Autodesk Fusion 360 part; units mm, degrees
sketch "Sketch1" plane through (0, 0, 0) normal (0, 0, 1) x (1, 0, 0)
  line L0 (0, 0) -> (74, 0)
  line L1 (74, 0) -> (74, 83)
  line L2 (74, 83) -> (0, 83)
  line L3 (0, 83) -> (0, 0)
  dimension "d1" = 74
  dimension "d2" = 83
extrude "Extrude1" add sketch "Sketch1" along normal blind 5
sketch "Sketch2" plane through (0, 0, 5) normal (0, 0, 1) x (-1, 0, 0)
  line L0 (0, -83) -> (0, 0)
  line L1 (0, 0) -> (-74, 0)
  line L2 (-74, 0) -> (-74, -83)
  line L3 (-74, -83) -> (0, -83)
  line L4 (-30.5, -77.2) -> (-71, -77.2)
  line L5 (-71, -77.2) -> (-71, -42.5)
  line L6 (-71, -42.5) -> (-30.5, -42.5)
  line L7 (-30.5, -42.5) -> (-30.5, -77.2)
  line L8 (-55.8, -22.25) -> (-67.8, -22.25)
  line L9 (-67.8, -22.25) -> (-67.8, -10.25)
  line L10 (-67.8, -10.25) -> (-55.8, -10.25)
  line L11 (-55.8, -10.25) -> (-55.8, -22.25)
  line L12 (-55.8, -35.25) -> (-67.8, -35.25)
  line L13 (-67.8, -35.25) -> (-67.8, -23.25)
  line L14 (-67.8, -23.25) -> (-55.8, -23.25)
  line L15 (-55.8, -23.25) -> (-55.8, -35.25)
  line L16 (-55.8, -29.25) -> (-67.8, -29.25) construction
  line L17 (-61.8, -35.25) -> (-61.8, -23.25) construction
  circle A0 centre (-61.8, -29.25) radius 5
  line L18 (-61.8, -22.25) -> (-61.8, -10.25) construction
  line L19 (-55.8, -16.25) -> (-67.8, -16.25) construction
  circle A1 centre (-61.8, -16.25) radius 5
  line L20 (-25.25, -10.5) -> (-13.25, -10.5)
  line L21 (-13.25, -10.5) -> (-13.25, -22.5)
  line L22 (-13.25, -22.5) -> (-25.25, -22.5)
  line L23 (-25.25, -22.5) -> (-25.25, -10.5)
  circle A2 centre (-19.25, -16.5) radius 5
  line L24 (-38.8, -4) -> (-26.8, -4)
  line L25 (-26.8, -4) -> (-26.8, -16)
  line L26 (-26.8, -16) -> (-38.8, -16)
  line L27 (-38.8, -16) -> (-38.8, -4)
  circle A3 centre (-32.8, -10) radius 5
  line L28 (-38.8, -17) -> (-26.8, -17)
  line L29 (-26.8, -17) -> (-26.8, -29)
  line L30 (-26.8, -29) -> (-38.8, -29)
  line L31 (-38.8, -29) -> (-38.8, -17)
  circle A4 centre (-32.8, -23) radius 5
  line L32 (-53, -10.5) -> (-41, -10.5)
  line L33 (-41, -10.5) -> (-41, -22.5)
  line L34 (-41, -22.5) -> (-53, -22.5)
  line L35 (-53, -22.5) -> (-53, -10.5)
  circle A5 centre (-47, -16.5) radius 5
  line L36 (-14.75, -36.25) -> (-2.75, -36.25)
  line L37 (-2.75, -36.25) -> (-2.75, -48.25)
  line L38 (-2.75, -48.25) -> (-14.75, -48.25)
  line L39 (-14.75, -48.25) -> (-14.75, -36.25)
  circle A6 centre (-8.75, -42.25) radius 5
  line L40 (-14.75, -23.25) -> (-2.75, -23.25)
  line L41 (-2.75, -23.25) -> (-2.75, -35.25)
  line L42 (-2.75, -35.25) -> (-14.75, -35.25)
  line L43 (-14.75, -35.25) -> (-14.75, -23.25)
  circle A7 centre (-8.75, -29.25) radius 5
  circle A8 centre (-25.1, -55.75) radius 2.65
  dimension "d5" = 30.5
  dimension "d6" = 42.5
  dimension "d7" = 34.7
  dimension "d8" = 40.5
  dimension "d11" = 12
  dimension "d14" = 12
  dimension "d15" = 6.2
  dimension "d16" = 10.25
  dimension "d17" = 6.2
  dimension "d19" = 1
  dimension "d20" = 10
  dimension "d21" = 10
  dimension "d22" = 12
  dimension "d23" = 10
  dimension "d24" = 12
  dimension "d25" = 10
  dimension "d26" = 12
  dimension "d27" = 10
  dimension "d28" = 12
  dimension "d29" = 10
  dimension "d32" = 10.5
  dimension "d33" = 6
  dimension "d34" = 6
  dimension "d35" = 4
  dimension "d36" = 6
  dimension "d37" = 6
  dimension "d38" = 21
  dimension "d39" = 17
  dimension "d40" = 6
  dimension "d41" = 6
  dimension "d42" = 35.2
  dimension "d43" = 6
  dimension "d44" = 6
  dimension "d45" = 13.25
  dimension "d46" = 10.5
  dimension "d47" = 12
  dimension "d48" = 10
  dimension "d49" = 6
  dimension "d50" = 6
  dimension "d51" = 12
  dimension "d52" = 10
  dimension "d53" = 6
  dimension "d54" = 6
  dimension "d55" = 2.75
  dimension "d56" = 23.25
  dimension "d57" = 1
  dimension "d58" = 5.3
  dimension "d59" = 27.25
  dimension "d60" = 25.1
extrude "Extrude3" cut sketch "Sketch2" against normal blind 5 contours A8
extrude "Extrude2" cut sketch "Sketch2" against normal blind 5 contours L4 L5 L6 L7 | A0 | A1 | A2 | A3 | A4 | A5 | A6 | A7
sketch "Sketch3" plane through (74, 0, 0) normal (1, 0, 0) x (0, 1, 0)
  line L0 (0, 0) -> (83, 0)
  line L1 (83, 0) -> (83, 5)
  line L2 (83, 5) -> (0, 5)
  line L3 (0, 5) -> (0, 0)
  line L4 (0, 5) -> (7.4455, 5)
  line L5 (7.4455, 5) -> (7.4455, 0)
  line L6 (7.4455, 0) -> (0, 0)
  line L7 (0, 0) -> (0, 5)
  line L8 (15.1109, 0) -> (15.1109, 5)
  line L9 (15.1109, 5) -> (22.5564, 5)
  line L10 (22.5564, 5) -> (22.5564, 0)
  line L11 (22.5564, 0) -> (15.1109, 0)
  line L12 (30.2218, 0) -> (30.2218, 5)
  line L13 (30.2218, 5) -> (37.6673, 5)
  line L14 (37.6673, 5) -> (37.6673, 0)
  line L15 (37.6673, 0) -> (30.2218, 0)
  line L16 (45.3327, 0) -> (45.3327, 5)
  line L17 (45.3327, 5) -> (52.7782, 5)
  line L18 (52.7782, 5) -> (52.7782, 0)
  line L19 (52.7782, 0) -> (45.3327, 0)
  line L20 (60.4436, 0) -> (60.4436, 5)
  line L21 (60.4436, 5) -> (67.8891, 5)
  line L22 (67.8891, 5) -> (67.8891, 0)
  line L23 (67.8891, 0) -> (60.4436, 0)
  line L24 (75.5545, 0) -> (75.5545, 5)
  line L25 (75.5545, 5) -> (83, 5)
  line L26 (83, 5) -> (83, 0)
  line L27 (83, 0) -> (75.5545, 0)
  dimension "d70" = 7.4455
  dimension "d74" = 75.5545
  dimension "d75" = 0
extrude "Extrude4" add sketch "Sketch3" along normal blind 5 contours L0 L2 L3 L4 L5 L6 L7 | L0 L2 L8 L9 L10 L11 | L0 L2 L12 L13 L14 L15 | L0 L2 L16 L17 L18 L19 | L0 L2 L20 L21 L22 L23 | L0 L1 L2 L24 L25 L26 L27
sketch "Sketch4" plane through (0, 0, 0) normal (-1, 0, 0) x (0, -1, 0)
  line L0 (-83, 0) -> (0, 0)
  line L1 (0, 0) -> (0, 5)
  line L2 (0, 5) -> (-83, 5)
  line L3 (-83, 5) -> (-83, 0)
  line L4 (-83, 5) -> (-75.5545, 5)
  line L5 (-75.5545, 5) -> (-75.5545, 0)
  line L6 (-75.5545, 0) -> (-83, 0)
  line L7 (-83, 0) -> (-83, 5)
  line L8 (-67.8891, 0) -> (-67.8891, 5)
  line L9 (-67.8891, 5) -> (-60.4436, 5)
  line L10 (-60.4436, 5) -> (-60.4436, 0)
  line L11 (-60.4436, 0) -> (-67.8891, 0)
  line L12 (-52.7782, 0) -> (-52.7782, 5)
  line L13 (-52.7782, 5) -> (-45.3327, 5)
  line L14 (-45.3327, 5) -> (-45.3327, 0)
  line L15 (-45.3327, 0) -> (-52.7782, 0)
  line L16 (-37.6673, 0) -> (-37.6673, 5)
  line L17 (-37.6673, 5) -> (-30.2218, 5)
  line L18 (-30.2218, 5) -> (-30.2218, 0)
  line L19 (-30.2218, 0) -> (-37.6673, 0)
  line L20 (-22.5564, 0) -> (-22.5564, 5)
  line L21 (-22.5564, 5) -> (-15.1109, 5)
  line L22 (-15.1109, 5) -> (-15.1109, 0)
  line L23 (-15.1109, 0) -> (-22.5564, 0)
  line L24 (-7.4455, 0) -> (-7.4455, 5)
  line L25 (-7.4455, 5) -> (0, 5)
  line L26 (0, 5) -> (0, 0)
  line L27 (0, 0) -> (-7.4455, 0)
  dimension "d78" = 7.4455
  dimension "d81" = 75.5545
  dimension "d82" = 0
extrude "Extrude5" add sketch "Sketch4" along normal blind 5 contours L0 L2 L3 L4 L5 L6 L7 | L0 L2 L8 L9 L10 L11 | L0 L2 L12 L13 L14 L15 | L0 L2 L16 L17 L18 L19 | L0 L2 L20 L21 L22 L23 | L0 L1 L2 L24 L25 L26 L27
sketch "Sketch5" plane through (0, 0, 0) normal (0, -1, 0) x (1, 0, 0)
  line L0 (-5, 0) -> (79, 0)
  line L1 (79, 0) -> (79, 5)
  line L2 (79, 5) -> (-5, 5)
  line L3 (-5, 5) -> (-5, 0)
  line L4 (0, 5) -> (6.6273, 5)
  line L5 (6.6273, 5) -> (6.6273, 0)
  line L6 (6.6273, 0) -> (0, 0)
  line L7 (0, 0) -> (0, 5)
  line L8 (13.4745, 0) -> (13.4745, 5)
  line L9 (13.4745, 5) -> (20.1018, 5)
  line L10 (20.1018, 5) -> (20.1018, 0)
  line L11 (20.1018, 0) -> (13.4745, 0)
  line L12 (26.9491, 0) -> (26.9491, 5)
  line L13 (26.9491, 5) -> (33.5764, 5)
  line L14 (33.5764, 5) -> (33.5764, 0)
  line L15 (33.5764, 0) -> (26.9491, 0)
  line L16 (40.4236, 0) -> (40.4236, 5)
  line L17 (40.4236, 5) -> (47.0509, 5)
  line L18 (47.0509, 5) -> (47.0509, 0)
  line L19 (47.0509, 0) -> (40.4236, 0)
  line L20 (53.8982, 0) -> (53.8982, 5)
  line L21 (53.8982, 5) -> (60.5255, 5)
  line L22 (60.5255, 5) -> (60.5255, 0)
  line L23 (60.5255, 0) -> (53.8982, 0)
  line L24 (67.3727, 0) -> (67.3727, 5)
  line L25 (67.3727, 5) -> (74, 5)
  line L26 (74, 5) -> (74, 0)
  line L27 (74, 0) -> (67.3727, 0)
  point P0 (0, 5)
  dimension "d85" = 6.6273
  dimension "d88" = 67.3727
  dimension "d89" = 0
extrude "Extrude6" add sketch "Sketch5" along normal blind 5 contours L0 L2 L4 L5 L6 L7 | L0 L2 L8 L9 L10 L11 | L0 L2 L12 L13 L14 L15 | L0 L2 L16 L17 L18 L19 | L0 L2 L20 L21 L22 L23 | L0 L2 L24 L25 L26 L27
sketch "Sketch6" plane through (0, 83, 0) normal (0, 1, 0) x (-1, 0, 0)
  line L0 (-79, 0) -> (5, 0)
  line L1 (5, 0) -> (5, 5)
  line L2 (5, 5) -> (-79, 5)
  line L3 (-79, 5) -> (-79, 0)
  line L4 (-74, 5) -> (-67.3727, 5)
  line L5 (-67.3727, 5) -> (-67.3727, 0)
  line L6 (-67.3727, 0) -> (-74, 0)
  line L7 (-74, 0) -> (-74, 5)
  line L8 (-60.5255, 0) -> (-60.5255, 5)
  line L9 (-60.5255, 5) -> (-53.8982, 5)
  line L10 (-53.8982, 5) -> (-53.8982, 0)
  line L11 (-53.8982, 0) -> (-60.5255, 0)
  line L12 (-47.0509, 0) -> (-47.0509, 5)
  line L13 (-47.0509, 5) -> (-40.4236, 5)
  line L14 (-40.4236, 5) -> (-40.4236, 0)
  line L15 (-40.4236, 0) -> (-47.0509, 0)
  line L16 (-33.5764, 0) -> (-33.5764, 5)
  line L17 (-33.5764, 5) -> (-26.9491, 5)
  line L18 (-26.9491, 5) -> (-26.9491, 0)
  line L19 (-26.9491, 0) -> (-33.5764, 0)
  line L20 (-20.1018, 0) -> (-20.1018, 5)
  line L21 (-20.1018, 5) -> (-13.4745, 5)
  line L22 (-13.4745, 5) -> (-13.4745, 0)
  line L23 (-13.4745, 0) -> (-20.1018, 0)
  line L24 (-6.6273, 0) -> (-6.6273, 5)
  line L25 (-6.6273, 5) -> (0, 5)
  line L26 (0, 5) -> (0, 0)
  line L27 (0, 0) -> (-6.6273, 0)
  point P0 (-74, 5)
  point P1 (-67.3727, 0)
  dimension "d94" = 67.3727
  dimension "d95" = 0
extrude "Extrude7" add sketch "Sketch6" along normal blind 5 contours L0 L2 L4 L5 L6 L7 | L0 L2 L8 L9 L10 L11 | L0 L2 L12 L13 L14 L15 | L0 L2 L16 L17 L18 L19 | L0 L2 L20 L21 L22 L23 | L0 L2 L24 L25 L26 L27
equation "pikkus = 83 mm"
equation "laius = 74 mm"
equation "paksus = 5 mm"
equation "pikkus_tapp = pikkus / 11 - 0.1 mm"
equation "laius_tapp = laius / 11 - 0.1 mm"
equation "d70 = pikkus_tapp"
equation "d74 = pikkus - pikkus_tapp"
equation "d76 = paksus"
equation "d78 = pikkus_tapp"
equation "d81 = pikkus - pikkus_tapp"
equation "d83 = paksus"
equation "d85 = laius_tapp"
equation "d88 = laius - laius_tapp"
equation "d90 = paksus"
equation "d94 = laius - laius_tapp"
equation "d96 = paksus"
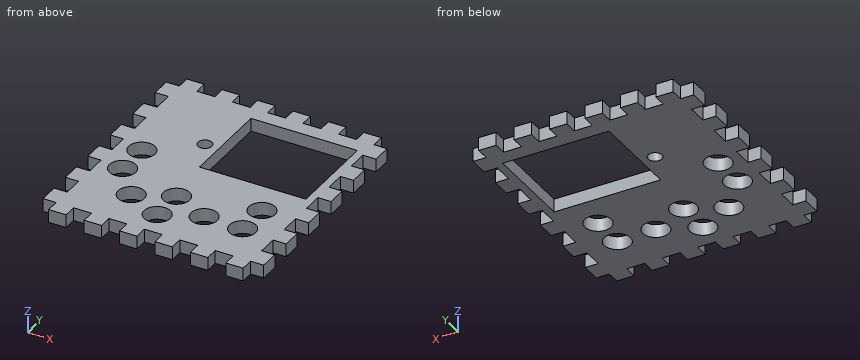
Can you work these out from the model? Positions are in its coordinate system, mm. Give positions to 0.01 mm unless a question says otherwise; leave off trailing zeros. Write each loop counter-clockwise with the first axis right and the second up, starting at its lowest first coordinate (ties: lowest second). Pieces come first, ordered by that corner, then holes. Notation, with made-up numbers: M 62.25,45.25 L 70.25,45.25 A35 cw 70.25,83.25 Z; hole C 2,77 d10. An arc over 180 degrees is marked long. Answer in a Markdown table with one row per item. Add a question column.
Item 1: For pin 1 Ø1.5 at (x, z) = (76.5, 3) entering from +Y; pin 2 Ø10 at (x, y) = (29.5, 31.5) entering from -Z; pin 3 Ø2 at (x, y) = (62, 31.5) entering from -Z; pin 4 Ø1.5 at (y, z) = (-1.5, 2) entering from +X, each with a flat end and sliding along its axis, tell me the tip position at first contact or that it passes through.
Item 2: Imagine slicing it at A-A, the plane x = 61.8. Write out the boundary of the cut face in (y, z).
Item 3: Imagine slicing it at D-D, the plane y = 10. Write out the boundary of the cut face in (x, z).
Item 4: Imagine slicing it at C-C, the plane x = 8.75. Write out the boundary of the cut face in (y, z).
Item 5: Please list where these lines run through material, in increasing order: L1, parallel to X at y = 16.25, z = 1.1; L2, parallel to X at y = 55.75, z = 3.35; L3, parallel to X at y = 29.25, z = 3.7.
Item 6: Imagine slicing it at B-B, the plane y = 70. Write out the boundary of the cut face in (x, z).
Evaluation:
| question | item | result |
|---|---|---|
| 1 | pin 1 | stops at y = 83 |
| 1 | pin 2 | stops at z = 0 |
| 1 | pin 3 | passes through |
| 1 | pin 4 | stops at x = 74 |
| 2 | outline | M 0,0 L 11.25,0 L 11.25,5 L 0,5 Z; M 21.25,0 L 24.25,0 L 24.25,5 L 21.25,5 Z; M 34.25,0 L 42.5,0 L 42.5,5 L 34.25,5 Z; M 77.2,0 L 83,0 L 83,5 L 77.2,5 Z |
| 3 | outline | M 0,0 L 27.8,0 L 27.8,5 L 0,5 Z; M 37.8,0 L 74,0 L 74,5 L 37.8,5 Z |
| 4 | outline | M 0,0 L 24.25,0 L 24.25,5 L 0,5 Z; M 34.25,0 L 37.25,0 L 37.25,5 L 34.25,5 Z; M 47.25,0 L 83,0 L 83,5 L 47.25,5 Z |
| 5 | L1 | x = -5 to 14.26, 24.24 to 42.01, 51.99 to 56.8, 66.8 to 79 |
| 5 | L2 | x = 0 to 22.45, 27.75 to 30.5, 71 to 74 |
| 5 | L3 | x = 0 to 3.75, 13.75 to 56.8, 66.8 to 74 |
| 6 | outline | M 0,0 L 30.5,0 L 30.5,5 L 0,5 Z; M 71,0 L 74,0 L 74,5 L 71,5 Z |
